Input: part model. Units: mm. Frame: model coordinates. Face numbers are marked on the shaded views. Coordinates: 2 decimals unless noted, no trailing zeros. Write each loop counter-clockwise with the first axis right and the second up, starting at its lowest first coordinate (ties: lowest second). Pieces come first, ordered by that corner, then holes. Notation, with made-up numbers: M 75.25,30.25 L 112.25,30.25 A27 ccw 112.25,64.25 Z; hole C 0.25,49 d11. An arc over 180 degrees is marked long. Use one line per item in the form item = value.
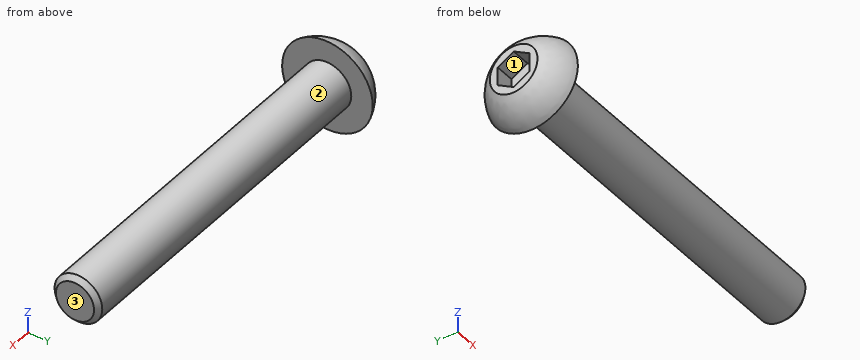
from build123d import *

# Parameters (mm, degrees)
CHAMFER1_SIZE      = 0.3
CUT_EXTRUDE1_DEPTH = 1.2


with BuildPart() as part:
    # Sketch1 → Revolve1 (revolve)
    with BuildSketch(Plane(origin=(0, 0, 0), x_dir=(1, 0, 0), z_dir=(0, 1, 0))):
        with BuildLine():
            ThreePointArc((3.937869631, 1.510997792), (3.937864578, 1.505498886), (3.937849421, 1.5))
            Line((3.937849421, 1.5), (22, 1.5))
            Line((22, 1.5), (22, 3))
            Line((22, 3), (3.541094523, 3))
            ThreePointArc((3.541094523, 3), (3.836974876, 2.281477847), (3.937869631, 1.510997792))
        make_face()
        with BuildLine():
            Line((0, 3), (0, 1.5))
            Line((0, 1.5), (3.937849421, 1.5))
            ThreePointArc((3.937849421, 1.5), (3.937864578, 1.505498886), (3.937869631, 1.510997792))
            ThreePointArc((3.937869631, 1.510997792), (3.836974876, 2.281477847), (3.541094523, 3))
            Line((3.541094523, 3), (0, 3))
        make_face()
        with BuildLine():
            Line((-1.65, 1.5), (0, 1.5))
            Line((0, 1.5), (0, 3))
            Line((0, 3), (0, 4.35))
            ThreePointArc((0, 4.35), (-0.949304344, 3.826927531), (-1.65, 3))
            Line((-1.65, 3), (-1.65, 2.5))
            Line((-1.65, 2.5), (-1.65, 1.5))
        make_face()
    revolve(axis=Axis((0, 0, -1.5), (1, 0, 0)))

    # Chamfer1
    chamfer1_edges = [part.edges().sort_by_distance(p)[0] for p in [
        (22, 0, 0),
    ]]
    chamfer(chamfer1_edges, length=CHAMFER1_SIZE)

    # Sketch2 → Cut-Extrude1 (cut)
    with BuildSketch(Plane.ZY.offset(1.65)):
        Polygon((-0.345299462, 0), (-0.922649731, 1), (-2.077350269, 1), (-2.654700538, 0), (-2.077350269, -1), (-0.922649731, -1), align=None)
    extrude(amount=-CUT_EXTRUDE1_DEPTH, mode=Mode.SUBTRACT)


solid = part.part
(1) Line query: probe 1 along X at (y, z) = (1.3, 0.45); probe 2 along Y at (x, z) = (3, -1.55); probe 3 along Y at (x, z) = (17.5, -2.4). Output: solid intervals per line, ascending.
Computed:
probe_1 = -0.93 to 0
probe_2 = -1.5 to 1.5
probe_3 = -1.2 to 1.2
(2) First-contact query: pin 1 Ø0.9 at (x, z) = (-1, -1.5) entering from -Y; pin 2 Ø0.9 at (x, z) = (-1, -1.5) entering from +Y; pin 3 Ø1 at (x, y) = (13.5, -1.5) entering from -Z. Flat tips, straight axial feed; report the tip coordinate or a pass-through.
Computed:
pin_1 = -2.6
pin_2 = 2.6
pin_3 = -2.62
(3) Section query A-A on x = 14. Return the cut outline in (y, z).
Computed:
outline = C 0,-1.5 d3
(4) Pull-direction query (Y, two-part tool) for the marked faces 1, 2 and 3; classes: pulls with the +Y half, pulls with the -Y half, needs draft (parallel to the pull), parting line crosses it, or undercut.
Computed:
face_1 = undercut
face_2 = parting line crosses it
face_3 = needs draft
